from build123d import *

# Parameters (mm, degrees)
F0_W     = 50
F0_H     = 20
F1_DEPTH = 6
F2_W     = 13
F2_H     = 1.5
F3_DEPTH = 18.4
F4_R     = 1


with BuildPart() as f1:
    # F0 (on Top) → F1 (new body)
    with BuildSketch(Plane.XY):
        with Locations((25, 10)):
            Rectangle(F0_W, F0_H)
    extrude(amount=F1_DEPTH)

    # F2 (on face) → F3 (cut, through all)
    with BuildSketch(Plane.XZ):
        Polygon((18.5, 4.5), (16.35, 4.5), (16.35, 1.9), (33.65, 1.9), (33.65, 4.5), (31.5, 4.5), align=None)
        with Locations((25, 5.25)):
            Rectangle(F2_W, F2_H)
    extrude(amount=-F3_DEPTH, mode=Mode.SUBTRACT)

    # F4
    f4_edges = [f1.edges().sort_by_distance(p)[0] for p in [
        (50, 10, 6),
        (50, 10, 0),
        (0, 10, 0),
        (0, 10, 6),
    ]]
    fillet(f4_edges, radius=F4_R)


solid = f1.part
Can you work these out from the model? Positions are in its coordinate system, mm. A direction names the side the tool comes from. Give positions to 0.01 mm unless a question says otherwise; leave off trailing zeros. Loops run counter-clockwise (first coordinate to the right, second up) from the corner with the lowest first, then second, coordinate; pieces in that order, holes last. Notation, with made-up numbers: M 1.25,2.25 L 13.25,2.25 A21 ccw 13.25,12.25 Z; hole C 51,-15 d10. An arc over 180 degrees is marked long. One line per item, written item: value. Start each with the question number.
1) On a 3-axis mill with a long thin cutter (end or side, diameter ignored), from which of +Z, -Z, +X, -X, +Y, -Y can I reach the whole of each face in a straight line? I mean faces 4 (the face through (0.285, 10.14, 5.699)), 5 (the face through (16.35, 9, 3)), 6 (the face through (31.5, 9, 5)). Say none if no direction works.
2) Thinking about a two-plate mould opening in X: for faces 1 (the face through (24.7, 0, 1.6)), 2 (the face through (18.5, 9, 5)), 3 (the face through (0, 10, 3)), which applies, +X half, -X half, draft (parallel to the pull), parting line (faces both ways), or undercut?
3) If we section it at A-A, the plane x = 17.5: Write out the boundary of the cut face in (y, z), and give its area (3 significant figures).
4) I'm going to push a flat-ended pin straight in: pin 1 (1.2 mm diameter, centred on x = 21.5, z = 3.5, fed in from -Y). Where does the tip first touch, or does it pass through?
5) If we section it at C-C, the plane z = 3.05: Write out the boundary of the cut face in (x, y).
6) If I drill on line 1 (X direction, y = 11.75, z = 2.8); line 2 (Z direction, x = 22, y = 4.75); line 3 (Y direction, x = 29.5, z = 5.45), over which ranges is the centre line in solid material (lowest first)? Write a range as [from, to].
7) If we section it at B-B, the plane y = 11.75: Write out the boundary of the cut face in (x, z).
8) If we section it at D-D, the plane x = 23.5: Write out the boundary of the cut face in (y, z).
Completed:
1. face 4: +Z, -X, +Y, -Y
1. face 5: -Y
1. face 6: +Z, -Y
2. face 1: draft
2. face 2: undercut
2. face 3: -X half
3. outline: M 0,0 L 20,0 L 20,6 L 0,6 L 0,4.5 L 18.4,4.5 L 18.4,1.9 L 0,1.9 Z
3. area: 72.2 mm^2
4. pin 1: stops at y = 18.4
5. outline: M 0,0 L 16.35,0 L 16.35,18.4 L 33.65,18.4 L 33.65,0 L 50,0 L 50,20 L 0,20 Z
6. line 1: x = [0, 16.35], [33.65, 50]
6. line 2: z = [0, 1.9]
6. line 3: y = [18.4, 20]
7. outline: M 0,1 A1 ccw 1,0 L 49,0 A1 ccw 50,1 L 50,5 A1 ccw 49,6 L 31.5,6 L 31.5,4.5 L 33.65,4.5 L 33.65,1.9 L 16.35,1.9 L 16.35,4.5 L 18.5,4.5 L 18.5,6 L 1,6 A1 ccw 0,5 Z
8. outline: M 0,0 L 20,0 L 20,6 L 18.4,6 L 18.4,1.9 L 0,1.9 Z
